Model file for the job. Use its own axes, mm. Face numbers are marked on the shaded views. A direction names the side the tool comes from. Coordinates: 2 decimals unless noted, no trailing zeros. Loops run counter-clockwise (first coordinate to the right, second up) from the corner with the lowest first, then second, coordinate; pieces in that order, holes last.
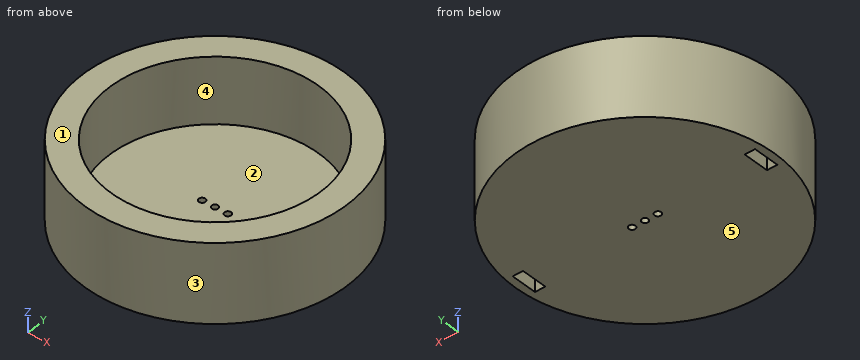
from build123d import *

# Parameters (mm, degrees)
F0_R     = 10
F0_R_2   = 8
F1_DEPTH = 6
F2_R     = 10
F2_W     = 0.8
F2_H     = 2
F2_R_2   = 0.25
F3_DEPTH = 1
F4_DEPTH = 1.5


with BuildPart() as f1:
    # F0 (on Top) → F1 (new body)
    with BuildSketch(Plane.XY):
        Circle(F0_R)
        Circle(F0_R_2, mode=Mode.SUBTRACT)
    extrude(amount=F1_DEPTH)

    # F2 (on Top) → F3 (join)
    with BuildSketch(Plane.XY):
        Circle(F2_R)
        with Locations((-9, 0)):
            Rectangle(F2_W, F2_H, mode=Mode.SUBTRACT)
        with Locations((-1, 0)):
            Circle(F2_R_2, mode=Mode.SUBTRACT)
        Circle(F2_R_2, mode=Mode.SUBTRACT)
        with Locations((1, 0)):
            Circle(F2_R_2, mode=Mode.SUBTRACT)
        with Locations((9, 0)):
            Rectangle(F2_W, F2_H, mode=Mode.SUBTRACT)
    extrude(amount=F3_DEPTH)

    # F2 (on Top) → F4 (cut)
    with BuildSketch(Plane.XY):
        with Locations((9, 0)):
            Rectangle(F2_W, F2_H)
        with Locations((-9, 0)):
            Rectangle(F2_W, F2_H)
    extrude(amount=F4_DEPTH, mode=Mode.SUBTRACT)


solid = f1.part
Q1. Slice it at B-B (y = 0). List the corners of the cut face in (x, z), and give its area (3 significant figures).
Answers:
outline: (-10, 0) - (-9.4, 0) - (-9.4, 1.5) - (-8.6, 1.5) - (-8.6, 0) - (-1.25, 0) - (-1.25, 1) - (-8, 1) - (-8, 6) - (-10, 6) - close; (-0.75, 0) - (-0.25, 0) - (-0.25, 1) - (-0.75, 1) - close; (0.25, 0) - (0.75, 0) - (0.75, 1) - (0.25, 1) - close; (1.25, 0) - (8.6, 0) - (8.6, 1.5) - (9.4, 1.5) - (9.4, 0) - (10, 0) - (10, 6) - (8, 6) - (8, 1) - (1.25, 1) - close
area: 36.1 mm2
Q2. Flat gauge pins, fed straight in: P1, Ø2, axis at y = -7, z = 3.5, coming from the -X side; P2, Ø3, axis at y = 3, z = 3, coming from the -X side; P3, Ø0.6, axis at x = 9, y = 0, coming from the -Z side. Where does each tip first touch, or does it go through?
Answers:
P1: stops at x = -8
P2: stops at x = -9.89
P3: stops at z = 1.5
Q3. Which spindle directions (+Z, -Z, +X, -X, +Y, -Y) get a long thin tool onto all of the face, cutting with end or side? Do the marked faces 4 and 5. Say none if no direction does.
Answers:
face 4: +Z
face 5: -Z, +X, -X, +Y, -Y
Q4. Drill centre lines: line 1 (Y direction, x = 0, z = 3.5); line 2 (Y direction, x = 0, z = 0.4). Where is each one in solid material? Low to high.
Answers:
line 1: y = -10 to -8, 8 to 10
line 2: y = -10 to -0.25, 0.25 to 10
Q5. Mould opens along X. For the marked faces 1, 2 and 3 say: +X half, -X half, draft (parallel to the pull), parting line (faces both ways), or undercut.
Answers:
face 1: draft
face 2: undercut
face 3: parting line
Q6. Slice it at D-D (x = 7). List the corners of the cut face in (y, z), and give its area (3 significant figures).
Answers:
outline: (-7.14, 0) - (7.14, 0) - (7.14, 6) - (3.87, 6) - (3.87, 1) - (-3.87, 1) - (-3.87, 6) - (-7.14, 6) - close
area: 47.0 mm2
Q7. Slice it at A-A (x = 0). List the corners of the cut face in (y, z), and give its area (3 significant figures).
Answers:
outline: (-10, 0) - (-0.25, 0) - (-0.25, 1) - (-8, 1) - (-8, 6) - (-10, 6) - close; (0.25, 0) - (10, 0) - (10, 6) - (8, 6) - (8, 1) - (0.25, 1) - close
area: 39.5 mm2
Q8. Slice it at C-C (z = 3.3). List the corners of the cut face in (x, y).
Answers:
outline: circle Ø20 at (0, 0); hole circle Ø16 at (0, 0)
